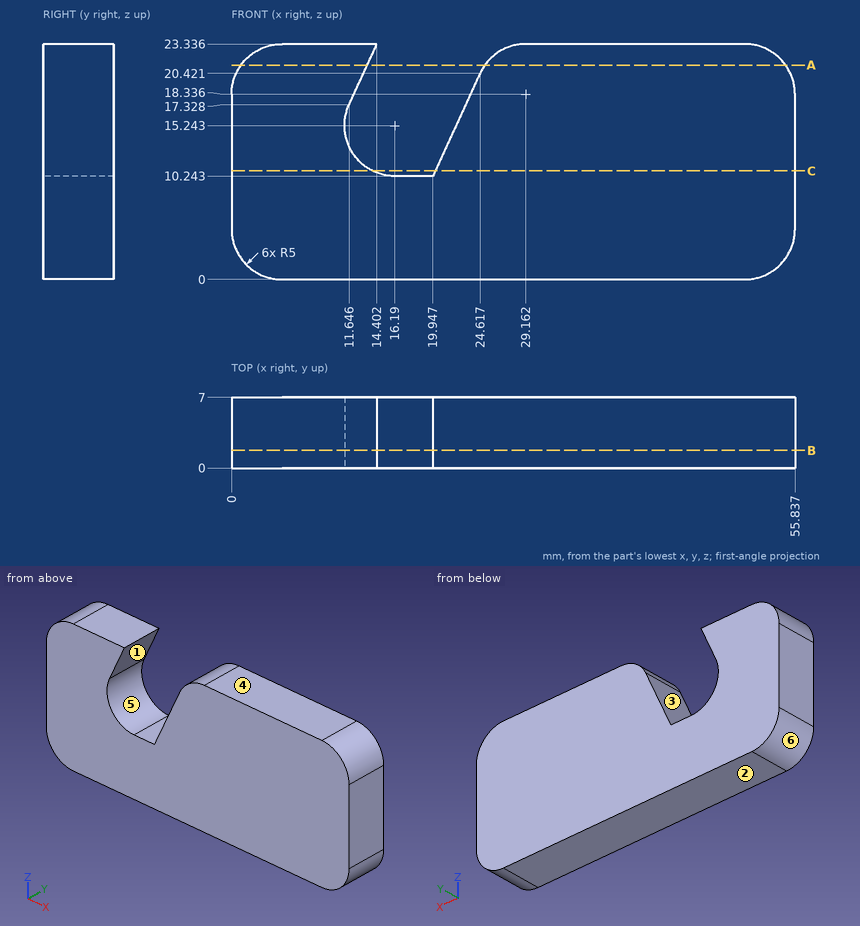
Could you check a few things on this drawing? It's one solid part, dimensions in mm from its lowest x, y, z. A direction names the side the tool comes from. Coordinates: 2 decimals unless noted, no trailing zeros. Order: outer loops, then holes, each group sorted by start corner. A loop starts at its lowest first (then second) coordinate and runs counter-clockwise, first axis right, second up.
1. If we section it at B-B (y = 1.75): Please give me the cut outline in (x, z) (1 decimal).
2. Thinking about a two-plate mould opening in Z: for the marked faces 4, 5 and 6, which applies, +Z half, -Z half, draft (parallel to the pull), parting line (faces both ways), or undercut?
3. If we section it at A-A (z = 21.25): Please give me the cut outline in (x, y) (1 decimal), then the cut area to 3 significant figures.
4. For the marked faces 1, 2 and 3, which set-ups out of +Z, -Z, +X, -X, +Y, -Y let a thin tool reach every point of the face, with its end or its side?
5. I need wall thicknesses on line 1 (X direction, y = 3.25, z = 21.25) (1 decimal); line 2 (X direction, y = 1, z = 12) (1 decimal); line 3 (Z direction, x = 18, y = 3.5). Which ranges of each line are inside material? Lowest first, please.
6. I'm going to push a flat-ended pin straight in: pin 1 (3 mm diameter, centred on x = 18, y = 3, fed in from +Z). Where does the tip first touch, or does it pass through?
7. If we section it at C-C (z = 10.75): Please give me the cut outline in (x, y).
Entries:
1. outline: (0, 5) arc R5 ccw to (5, 0) - (50.8, 0) arc R5 ccw to (55.8, 5) - (55.8, 18.3) arc R5 ccw to (50.8, 23.3) - (29.2, 23.3) arc R5 ccw to (24.6, 20.4) - (19.9, 10.2) - (16.2, 10.2) arc R5 cw to (11.6, 17.3) - (14.4, 23.3) - (5, 23.3) arc R5 ccw to (0, 18.3) - close
2. face 4: +Z half
2. face 5: undercut
2. face 6: -Z half
3. outline: (0.9, 0) - (13.4, 0) - (13.4, 7) - (0.9, 7) - close; (25.1, 0) - (54.9, 0) - (54.9, 7) - (25.1, 7) - close
3. area: 296 mm2
4. face 1: +Y, -Y
4. face 2: -Z, +X, -X, +Y, -Y
4. face 3: +Z, +Y, -Y
5. line 1: x = 0.9 to 13.4, 25.1 to 54.9
5. line 2: x = 0 to 12.4, 20.8 to 55.8
5. line 3: z = 0 to 10.24
6. pin 1: stops at z = 10.24
7. outline: (0, 0) - (14, 0) - (14, 7) - (0, 7) - close; (20.18, 0) - (55.84, 0) - (55.84, 7) - (20.18, 7) - close
